Could you check a few things on this model? Use its own coordinates, in mm. Face numbers are marked on the shaded views. A direction names the side the tool comes from. Give positions to 0.01 mm unless a question says otherwise; leave off trailing zeros. Order: outer loops, then holes, each group sorted by start corner. A loop starts at its lowest first (then second) coordinate and runs counter-clockwise, first axis right, second up. Notation, with made-up numbers: (30, 54) -> (87, 54) arc R21 ccw to (87, 61) -> close; hole circle Ø8 at (63.25, -37.5). An arc over 180 degrees is marked (long way). One line per item, written item: value.
```python
from build123d import *

# Parameters (mm, degrees)
SKETCH1_W           = 80
SKETCH1_H           = 54
BOSS_EXTRUDE2_DEPTH = 15.5
FILLET1_R           = 2
Y_WING_START        = -26.76167351
Y_WING_DEPTH        = 8
Y_WING_START_2      = -32.76167351
Y_WING_2_OUTLINE_R  = 2.5
Y_WING_2_DEPTH      = 6


with BuildPart() as part:
    # Sketch1 → Boss-Extrude2 (new body)
    with BuildSketch(Plane(origin=(0, 0, 0), x_dir=(1, 0, 0), z_dir=(0, 1, 0))):
        with Locations((40, 27)):
            Rectangle(SKETCH1_W, SKETCH1_H)
    extrude(amount=BOSS_EXTRUDE2_DEPTH)

    # Fillet1
    fillet1_edges = [part.edges().sort_by_distance(p)[0] for p in [
        (0, 7.75, -54),
        (80, 7.75, -54),
        (80, 7.75, 0),
        (0, 7.75, 0),
    ]]
    fillet(fillet1_edges, radius=FILLET1_R)


with BuildPart() as body_2:
    # Y-Wing: read off the stored shape, not the designer's step
    # Y-Wing outline → Y-Wing (new body)
    with BuildSketch(Plane(origin=(0, 0, 0), x_dir=(1, 0, 0), z_dir=(0, 1, 0)).offset(Y_WING_START)):
        Polygon((-37.998848216, 80.77793428), (-49.561243891, 80.77793428), (-51.452110178, 83.77793428), (-69.950345376, 80.625586413), (-69.950345376, 70.93293428), (-51.452110178, 67.77793428), (-49.561243891, 70.77793428), (-37.998848216, 70.77793428), (-37.998848216, 66.17793428), (-43.764531914, 66.17793428), (-43.764531914, 58.130000785), (-6.764531914, 58.130000785), (-6.764531914, 66.17793428), (-27.548546514, 66.17793428), (-27.548546514, 70.77793428), (-24.545586254, 70.77793428), (-24.545586254, 80.77793428), (-27.548546514, 80.77793428), (-27.548546514, 85.37793428), (-6.764531914, 85.37793428), (-6.764531914, 93.87793428), (-43.764531914, 93.87793428), (-43.764531914, 85.37793428), (-37.998848216, 85.37793428), align=None)
    extrude(amount=Y_WING_DEPTH)

    # Y-Wing 2 outline → Y-Wing 2 (add)
    with BuildSketch(Plane(origin=(0, 0, 0), x_dir=(1, 0, 0), z_dir=(0, 1, 0)).offset(Y_WING_START_2)):
        with Locations((-38.150345376, 75.778331613)):
            Circle(Y_WING_2_OUTLINE_R)
    extrude(amount=Y_WING_2_DEPTH)


with BuildPart() as body_2_1:
    # Body-Move/Copy3: moved
    add(body_2.part.moved(Location((81.260162004, 34.341820547, 49.133266847))))


with BuildPart() as part_1:
    add(part.part)

    # Intersect1: read off the stored shape, not the designer's step
    # Intersect1: cut body 2
    add(body_2_1.part, mode=Mode.SUBTRACT)


solid = part_1.part
```
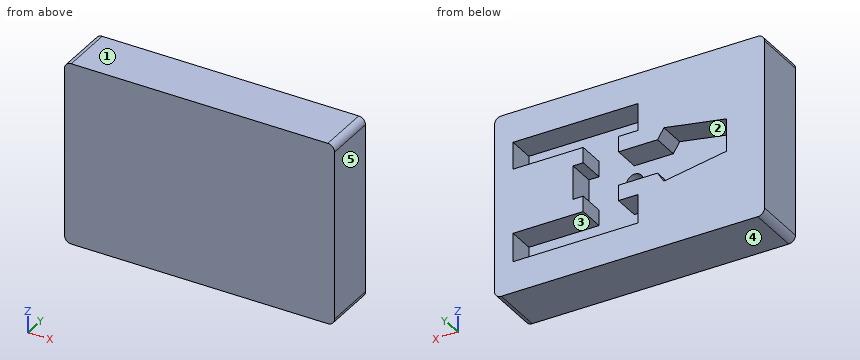
1) For P1, Ø2.5, axis at x = 44, z = -26.5, coming from the +Y side, with a flat end and sliding along its axis, tell me the tip position at first contact or that it passes through.
Answer below:
P1: stops at y = 1.58
2) Suppose I cut it at C-C, the plane x = 68. Write out the boundary of the cut face in (y, z), then the cut area to 3 significant figures.
Answer below:
outline: (0, -54) -> (15.5, -54) -> (15.5, -44.74) -> (7.58, -44.74) -> (7.58, -36.24) -> (15.5, -36.24) -> (15.5, -17.04) -> (7.58, -17.04) -> (7.58, -9) -> (15.5, -9) -> (15.5, 0) -> (0, 0) -> close
area: 706 mm2
3) For the marked faces 1 and 2, which set-ups out of +Z, -Z, +X, -X, +Y, -Y let a thin tool reach every point of the face, with its end or its side?
Answer below:
face 1: +Z, +X, -X, +Y, -Y
face 2: +Y
4) Suppose I cut it at D-D, the plane x = 21. Write out the boundary of the cut face in (y, z).
Answer below:
outline: (0, -54) -> (15.5, -54) -> (15.5, -33.14) -> (7.58, -33.14) -> (7.58, -20.15) -> (15.5, -20.15) -> (15.5, 0) -> (0, 0) -> close
5) If I drill on line 1 along Z through (x, y) = (67, 13); line 2 along X through (y, z) = (3, -26.5); line 3 along X through (y, z) = (13, -15), over which ranges is the centre line in solid material (lowest first)?
Answer below:
line 1: z = -54 to -44.74, -36.24 to -17.04, -9 to 0
line 2: x = 0 to 40.61, 45.61 to 80
line 3: x = 0 to 37.5, 74.5 to 80
6) We'd pull the mould along X, two halves only. Please class the marked faces 3, 4 and 5: +X half, -X half, draft (parallel to the pull), parting line (faces both ways), or undercut.
Answer below:
face 3: undercut
face 4: draft
face 5: +X half
7) Suppose I cut it at B-B, the plane x = 36.5. Write out the boundary of the cut face in (y, z).
Answer below:
outline: (0, -54) -> (15.5, -54) -> (15.5, -31.64) -> (7.58, -31.64) -> (7.58, -21.64) -> (15.5, -21.64) -> (15.5, 0) -> (0, 0) -> close
